Work out the finished part from the listing and answer in its coordinate system (mm). Face numbers are marked on the shaded views. A direction names the side the tool comes from. Round coordinates to 2 decimals unless told otherwise and drop trailing zeros. Order: outer loops, then holes, each group sorted by start corner. A loop starts at its lowest first (then second) coordinate and runs counter-clockwise, first axis right, second up. Notation, with made-up numbers: (-19.75, -30) - (-6.75, -30) arc R17 ccw to (-6.75, 0) - close; hole circle Ø2 at (86, 40.25). An arc over 180 degrees is marked (long way). Answer in a Markdown table with one row per item.
Autodesk Inventor part; units mm, degrees
ref_plane "YZ Plane" through (0, 0, 0) normal (1, 0, 0) x (0, 1, 0)
ref_plane "XZ Plane" through (0, 0, 0) normal (0, 1, 0) x (-1, 0, 0)
ref_plane "XY Plane" through (0, 0, 0) normal (0, 0, 1) x (1, 0, 0)
sketch "Base Profile" plane through (0, 0, 0) normal (0, 1, 0) x (-1, 0, 0)
  line L0 (0, 0) -> (13, 0)
  line L1 (13, 0) -> (13, -21.35)
  line L2 (13, -21.35) -> (0, -21.35)
  line L3 (0, -21.35) -> (0, 0)
  dimension "d407" = 13
  dimension "d408" = 21.35
extrude "Extrusion21" add sketch "Base Profile" along normal blind 33
sketch "Front Profile" plane through (0, 0, 0) normal (1, 0, 0) x (0, 0, -1)
  line L0 (0, 0) -> (21.35, 0)
  line L1 (21.35, 0) -> (21.35, 33)
  line L2 (0, 33) -> (21.35, 33)
  line L3 (0, 0) -> (0, 33)
  line L4 (0, 0) -> (0, 33)
  line L5 (0, 16.5) -> (15, 16.5)
  line L6 (15, 16.5) -> (15, 7.5)
  line L7 (15, 7.5) -> (0, 7.5)
  line L8 (0, 7.5) -> (0, 16.5)
  line L9 (15, 33) -> (15, 0)
  line L10 (21.35, 0) -> (21.35, 33)
  line L11 (21.35, 16.5) -> (15, 16.5) construction
  circle A0 centre (18.175, 29.825) radius 3.175
  circle A1 centre (18.175, 3.175) radius 3.175
  point P0 (0, 7.5)
  point P1 (18.175, 16.5)
  dimension "d411" = 6.35
  dimension "d412" = 7.5
  dimension "d413" = 9
extrude "Extrusion22" cut sketch "Front Profile" against normal through all contours L3 L5 L6 L7
hole "Hole27" at (0, 29.825, -18.175) at (0, 3.175, -18.175) direction (-1, 0, 0) diameter 2.459 end through all
fillet "Fillet4" radius 3.175 2 edges at (-6.5, 33, -21.35) (-6.5, 0, -21.35)
equation "\"extrusionWidth\" = 15"
equation "\"bearingOffsetFromBottom\" = 7.5"
equation "\"extrusionOffset\" = 33"
equation "\"bearingStackHeight\" = 9"
equation "\"bearingSlotLength\" = 5"
equation "\"bearingClearance\" = 13"
properties part number "A Idler" material "Aluminum 6061"
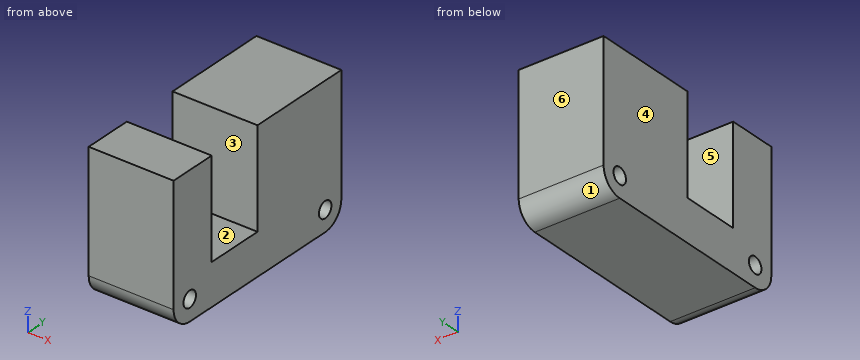
1) The mould has two halves that part along Y. Classify the marked faces 3, 4, 5 and 6: released by +Y, released by -Y, zero draft, split by the parting line, or undercut.
Filled in:
| item | result |
|---|---|
| face 3 | undercut |
| face 4 | zero draft |
| face 5 | undercut |
| face 6 | released by +Y |
2) Which of the six approach directions +Z, -Z, +X, -X, +Y, -Y give full straight-line access (tool end or side, diameter ignored) to the marked faces 1 and 2?
Filled in:
| item | result |
|---|---|
| face 1 | -Z, +X, -X, +Y |
| face 2 | +Z, +X, -X |
3) Find section D-D, the plane y = 14. Give the vertices of the cut face in (x, z).
Filled in:
| item | result |
|---|---|
| outline | (-13, -21.35) - (0, -21.35) - (0, -15) - (-13, -15) - close |
4) Find section A-A, the plane z = -2.75. Give the vertices of the cut face in (x, y).
Filled in:
| item | result |
|---|---|
| outline | (-13, 0) - (0, 0) - (0, 7.5) - (-13, 7.5) - close; (-13, 16.5) - (0, 16.5) - (0, 33) - (-13, 33) - close |
5) Find the intervals of material crossed by probe 1 along Y at (x, z) = (-9.25, -8); probe 2 along Y at (x, z) = (-3.5, -18); probe 3 along Z at (x, y) = (-5.75, 29), in increasing order. Write a range as from..to.
Filled in:
| item | result |
|---|---|
| probe 1 | y = 0..7.5, 16.5..33 |
| probe 2 | y = 0..1.96, 4.39..28.61, 31.04..33 |
| probe 3 | z = -21.35..-19.09, -17.26..0 |
6) Find section C-C, the plane z = -18.75. Give the vertices of the cut face in (x, y), then the cut area to 3 significant figures.
Filled in:
| item | result |
|---|---|
| outline | (-13, 0.05) - (0, 0.05) - (0, 2.09) - (-13, 2.09) - close; (-13, 4.26) - (0, 4.26) - (0, 28.74) - (-13, 28.74) - close; (-13, 30.91) - (0, 30.91) - (0, 32.95) - (-13, 32.95) - close |
| area | 371 mm^2 |
7) This flat-tipped pin is pushed along its axis until it touches: pin 1 (4.5 mm diameter, centred on x = -6, y = 13, fed in from +Z). Where does it stop, or does it pass through?
Filled in:
| item | result |
|---|---|
| pin 1 | stops at z = -15 |
8) Find section B-B, the plane x = -7. Give the number of separate pieces and of enclosed holes in the cut face, then the cut area to 3 significant figures.
Filled in:
| item | result |
|---|---|
| separate pieces | 1 |
| enclosed holes | 2 |
| area | 556 mm^2 |
